Work out the finished part from the listing and answer in its coordinate system (mm). Coordinates: 2 decimals unless noted, no trailing zeros. Order: outer loops, then holes, each group sorted by start corner. A loop starts at its lowest first (then second) coordinate and runs counter-clockwise, first axis right, second up.
```python
from build123d import *

# Parameters (mm, degrees)
SKETCH_R     = 50.164311
PAD_DEPTH    = 100
SKETCH001_R  = 47.549829
POCKET_DEPTH = 100.001


with BuildPart() as part:
    # Sketch → Pad (new body)
    with BuildSketch(Plane.XY):
        Circle(SKETCH_R)
    extrude(amount=PAD_DEPTH)

    # Sketch001 (on Face3 of Pad) → Pocket (cut, through all)
    with BuildSketch(Plane.XY.offset(100)):
        Circle(SKETCH001_R)
    extrude(amount=-POCKET_DEPTH, mode=Mode.SUBTRACT)

    # Sketch003 → SubtractiveLoft section 0
    with BuildSketch(Plane.XZ.offset(51)):
        Polygon((9.990768, 70), (-10.009232, 70), (-20.009232, 52.679492), (-10.009232, 35.358984), (9.990768, 35.358984), (19.990768, 52.679492), align=None)
    # Sketch004 → SubtractiveLoft section 1
    with BuildSketch(Plane.XZ.offset(-51)):
        Polygon((20, 52.685847), (10, 70.006355), (-10, 70.006355), (-20, 52.685847), (-10, 35.365339), (10, 35.365339), align=None)
    loft(ruled=True, mode=Mode.SUBTRACT)


solid = part.part
```
1. The part is cut by section B-B (x = 35.5). Determine the outline of the cut face in (y, z), plus the area to 3 significant figures.
2. The part is cut by section C-C (z = 30). Determine the outline of the cut face in (x, y), plus the area to 3 significant figures.
3. Flat-ended cylindrical pins translate along their axes: pin 1 (1.5 mm diameter, centred on y = 30, z = 73, fed in from +X); pin 2 (4 mm diameter, centred on x = -13, z = 42.5, fed in from -Y); pin 3 (1 mm diameter, centred on y = -9.5, z = 28, fed in from +X). Find the tip coordinate at first contact, or state that the pin passes through.
4. The part is cut by section A-A (y = 0). Determine the outline of the cut face in (x, z).
5. The part is cut by section D-D (x = 5). Count the separate pieces of the cut face and the enclosed holes in it, plus the area to 3 significant figures.
6. The mould has two halves that part along X. Classify faces 1 (the cylindrical face through (45.354, 14.283, 50.7)), 2 (the cylindrical face through (47.848, 15.068, 49.3)), 3 (the flat face through (44.4, -18.3, 100)): released by +X, released by -X, zero draft, split by the parting line, or undercut.
7. Consider probe 1 along Y at (x, z) = (0, 74); probe 2 along Y at (x, z) = (-29.5, 62). Determine where each line is inside the solid, lowest interval first.
Worked out:
1. outline: (-35.44, 0) - (-31.63, 0) - (-31.63, 100) - (-35.44, 100) - close; (31.63, 0) - (35.44, 0) - (35.44, 100) - (31.63, 100) - close
1. area: 762 mm2
2. outline: circle Ø100.33 at (0, 0); hole circle Ø95.1 at (0, 0)
2. area: 803 mm2
3. pin 1: stops at x = 40.75
3. pin 2: stops at y = -48.46
3. pin 3: stops at x = 49.35
4. outline: (-50.16, 0) - (-47.55, 0) - (-47.55, 100) - (-50.16, 100) - close; (47.55, 0) - (50.16, 0) - (50.16, 100) - (47.55, 100) - close
5. separate pieces: 4
5. enclosed holes: 0
5. area: 344 mm2
6. face 1: undercut
6. face 2: split by the parting line
6. face 3: zero draft
7. probe 1: y = -50.16 to -47.55, 47.55 to 50.16
7. probe 2: y = -40.57 to -37.29, 37.29 to 40.57
